Solid Edge part; units mm, degrees
sketch "Sketch1" plane through (0, 0, 0) normal (0, -1, 0) x (1, 0, 0)
  circle A0 centre (0, 0) radius 5
  line L0 (0, 7) -> (68.0003, 7)
  line L1 (0, -7) -> (68.0003, -7)
  arc A1 (0, -7) -> (0, 7) centre (0, 0) cw
  arc A2 (68.0003, 7) -> (68.0003, -7) centre (68.0003, 0) cw
  circle A3 centre (68.0003, 0) radius 5
extrude "Protrusion1" add sketch "Sketch1" along normal mid plane 11
fillet "Redondeo_1" [suppressed]
sketch "Sketch2" plane through (34.0002, 0, 0) normal (0, -1, 0) x (1, 0, 0)
  line L0 (-22.0002, -7) -> (0, 7)
  line L1 (-34.0002, -7) -> (-22.0002, -7)
  arc A0 (-34.0002, -7) -> (-34.0002, 7) centre (-34.0002, 0) cw
  line L2 (0, 7) -> (-34.0002, 7)
  dimension "D1" = 34.0002
  dimension "D2" = 34.0002
extrude "Cutout1" cut sketch "Sketch2" along normal mid plane 5
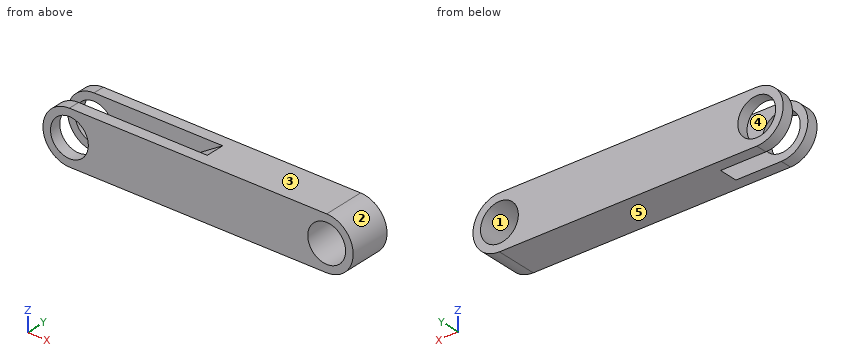
Here's how the part is built. I have some questions about the finished solid (model axes, mm). Face numbers are marked on the shaded views. A direction names the side the tool comes from. Round coordinates to 2 decimals unless told otherwise and drop trailing zeros. Order: outer loops, then holes, each group sorted by start corner. A loop starts at its lowest first (then second) coordinate and runs counter-clockwise, first axis right, second up. Notation, with made-up numbers: (2.5, 5.25) -> (40.5, 5.25) arc R19 ccw to (40.5, 22.25) -> close; hole circle Ø3 at (70, -23). An arc over 180 degrees is marked (long way). Return JSON: item names as keys, results as strings.
Q1. If we mould it in two halves opening along X, with no side actions, what happens to the marked faces 1, 2 and 3? For each: released by +X, released by -X, zero draft, split by the parting line, or undercut.
Filled sheet:
{"face 1": "undercut", "face 2": "released by +X", "face 3": "zero draft"}
Q2. If we section it at A-A on x = 10: List the corners of the cut face in (y, z) for me.
Filled sheet:
{"outline": "(-5.5, -7) -> (-2.5, -7) -> (-2.5, 7) -> (-5.5, 7) -> close; (2.5, -7) -> (5.5, -7) -> (5.5, 7) -> (2.5, 7) -> close"}
Q3. If we section it at C-C on y = -4.5: List the corners of the cut face in (x, z) for me, plus the area to 3 significant figures.
Filled sheet:
{"outline": "(0, -7) -> (68, -7) arc R7 ccw to (68, 7) -> (0, 7) arc R7 ccw to start; hole circle Ø10 at (0, 0); hole circle Ø10 at (68, 0)", "area": "949 mm^2"}
Q4. I need wall thicknesses on line 1 along Z through (x, y) = (0, -3.5); line 2 along Y through (x, z) = (12, 3.75); line 3 along Z through (x, y) = (-3.5, -3.5). Which ranges of each line are inside material? Lowest first, please. Write a range as from..to.
Filled sheet:
{"line 1": "z = -7..-5, 5..7", "line 2": "y = -5.5..-2.5, 2.5..5.5", "line 3": "z = -6.06..-3.57, 3.57..6.06"}
Q5. If we section it at D-D on y = -1.5: List the corners of the cut face in (x, z) for me.
Filled sheet:
{"outline": "(12, -7) -> (68, -7) arc R7 ccw to (68, 7) -> (34, 7) -> close; hole circle Ø10 at (68, 0)"}
Q6. Which directions (+Z, -Z, +X, -X, +Y, -Y) give clear straight access to the entire face, cutting with the end or side of a thin tool? Please do the marked faces 4 and 5.
Filled sheet:
{"face 4": "+Z, -X", "face 5": "-Z, +X, -X, +Y, -Y"}
Q7. For pin 1 Ø5 at (y, z) = (3, -4.5) entering from +X; pin 2 Ø8 at (x, z) = (0, 0) entering from +Y; pin 3 Ø1.5 at (x, y) = (11.5, 0) entering from +Z, each with a flat end and sliding along its axis, tell me the tip position at first contact or that it passes through.
Filled sheet:
{"pin 1": "stops at x = 74.71", "pin 2": "passes through", "pin 3": "stops at z = -6.84"}
Q8. If we section it at B-B on z = 0: List the corners of the cut face in (x, y) for me, plus the area to 3 significant figures.
Filled sheet:
{"outline": "(-7, -5.5) -> (-5, -5.5) -> (-5, -2.5) -> (-7, -2.5) -> close; (-7, 2.5) -> (-5, 2.5) -> (-5, 5.5) -> (-7, 5.5) -> close; (5, -5.5) -> (63, -5.5) -> (63, 5.5) -> (5, 5.5) -> (5, 2.5) -> (23, 2.5) -> (23, -2.5) -> (5, -2.5) -> close; (73, -5.5) -> (75, -5.5) -> (75, 5.5) -> (73, 5.5) -> close", "area": "582 mm^2"}
